Can you work these out from the model? Positions are in its coordinate system, mm. A direction names the side the tool comes from. Coordinates: 2 decimals unless noted, no trailing zeros. Order: outer loops, then holes, each group sorted by start corner. A loop starts at its lowest first (then second) coordinate and runs counter-clockwise, first axis right, second up. Notation, with made-up numbers: (-22.75, -1.75) - (25.25, -1.75) arc R13 cw to (25.25, 13.25) - close; hole circle Ø3 at (70.25, 34). An arc over 180 degrees is marked (long way). Use a Markdown table: item, result. Add a question column.
(1) If I drill on L1, parallel to Y at x = -5.25, z = 46; L2, parallel to X at y = -4, z = 45; L3, parallel to X at y = 3.25, z = 46.5, over which ranges is the centre line in solid material (lowest first)? Write a range as [from, to].
(2) We'd pull the mould along Y, two halves only. Please class faces 1 (the flat face through (-10, 6, 30)), 2 (the flat face through (0, 10, 30)), 3 (the flat face through (-9, 2.65, 30)): pulls with the +Y half, pulls with the -Y half, needs draft (parallel to the pull), parting line crosses it, or undercut.
(3) On a 3-axis mill with a long thin cutter (end or side, diameter ignored), from which of +Z, -Z, +X, -X, +Y, -Y can I reach the whole of each face in a straight line? I mean faces 4 (the flat face through (-9, -2.65, 30)), 5 (the flat face through (-10, -6, 30)), 6 (the flat face through (-6, 4.25, 30)). Say none if no direction works.
(4) I want a section at B-B (z = 56). List the corners of the cut face in (x, y) for me.
(5) I want a section at A-A (x = -5). List the corners of the cut face in (y, z) for me, and give its area (4 significant figures).
(6) I want a section at C-C (y = 1). List the corners of the cut face in (x, z) for me.
Solid Edge part; units mm, degrees
sketch "Sketch1" plane through (0, 0, 0) normal (0, 0, 1) x (1, 0, 0)
  line L0 (-10, -10) -> (10, -10)
  line L1 (10, -10) -> (10, 10)
  line L2 (10, 10) -> (-10, 10)
  line L3 (-10, 10) -> (-10, 2.65)
  line L4 (-8.5, 2.65) -> (-10, 2.65)
  line L5 (-8.5, 4.25) -> (-8.5, 2.65)
  line L6 (-3.3, 4.25) -> (-8.5, 4.25)
  arc A0 (-3.3, 4.25) -> (-3.3, -4.25) centre (-8.5833, 0) cw
  line L7 (-8.5, -4.25) -> (-3.3, -4.25)
  line L8 (-8.5, -2.65) -> (-8.5, -4.25)
  line L9 (-10, -2.65) -> (-8.5, -2.65)
  line L10 (-10, -2.65) -> (-10, -10)
extrude "Protrusion1" add sketch "Sketch1" along normal blind 61
Answers follow:
| question | item | result |
|---|---|---|
| 1 | L1 | y = [-10, -4.25], [4.25, 10] |
| 1 | L2 | x = [-10, -8.5], [-3.11, 10] |
| 1 | L3 | x = [-10, -8.5], [-2.63, 10] |
| 2 | face 1 | needs draft |
| 2 | face 2 | pulls with the +Y half |
| 2 | face 3 | undercut |
| 3 | face 4 | +Z, -Z, -X |
| 3 | face 5 | +Z, -Z, -X, +Y, -Y |
| 3 | face 6 | +Z, -Z |
| 4 | outline | (-10, -10) - (10, -10) - (10, 10) - (-10, 10) - (-10, 2.65) - (-8.5, 2.65) - (-8.5, 4.25) - (-3.3, 4.25) arc R6.78 cw to (-3.3, -4.25) - (-8.5, -4.25) - (-8.5, -2.65) - (-10, -2.65) - close |
| 5 | outline | (-10, 0) - (-4.25, 0) - (-4.25, 61) - (-10, 61) - close; (4.25, 0) - (10, 0) - (10, 61) - (4.25, 61) - close |
| 5 | area | 701.5 mm² |
| 6 | outline | (-1.88, 0) - (10, 0) - (10, 61) - (-1.88, 61) - close |
